Could you check a few things on this model? Use its own coordinates, in mm. A direction names the side the tool comes from. Give positions to 0.01 mm unless a question says otherwise; leave off trailing zeros. Loops run counter-clockwise (first coordinate to the right, second up) from the corner with the lowest first, then second, coordinate; pieces in that order, holes last. Notation, with made-up numbers: M -1,-14.75 L 58,-14.75 A7 ccw 58,-8.75 Z; hole C 81.5,-31.75 d10. An arc over 180 degrees is marked long. Use a Markdown table: item, result. Add a question column.
1) If I drill on line 1 along Z through (x, y) = (1, -6.5); line 2 along Y through (x, z) = (-2.25, -1.5); line 3 along Y through (x, z) = (0.5, -3.5), over which ranges is the centre line in solid material (lowest first)? Write a range as [from, to].
2) Will these pins go through, and if not, where does the flat tip stop? pin 1 Ø3 at (x, y) = (-1.5, 1.5) entering from -Z; pin 2 Ø4 at (y, z) = (3.5, 9) entering from +X; pin 3 Ø4 at (x, z) = (2, -4) entering from -Y; pin 4 Ø2 at (x, y) = (-4.5, 6) entering from -Z.
3) We'd pull the mould along X, two halves only. Please class faces 3 (the conical face through (-3.45, 2.65, 2.83)), 4 (the cylindrical face through (-1.19, 5.37, -0.13)), 5 (the flat face through (-5, 0, -9)): +X half, -X half, draft (parallel to the pull), parting line (faces both ways), or undercut.
4) Which directions (+Z, -Z, +X, -X, +Y, -Y) give clear straight access to the entire face, cutting with the end or side of a thin tool? Please do faces 1 (the cylindrical face through (7.81, 1.73, 11.71)), 2 (the flat face through (1.7, 5.4, 9)).
5) Suppose I cut it at A-A on z = -3.25. List the corners of the cut face in (x, y) for me, and give its area (3 significant figures).
6) Suppose I cut it at B-B on z = 5. List the corners of the cut face in (x, y) for me, and give its area (3 significant figures).
Solid Edge part; units mm, degrees
sketch "Sketch1" plane through (0, 0, 0) normal (0, 0, 1) x (1, 0, 0)
  circle A0 centre (0, 0) radius 5.5
extrude "Ajout_matière_1" add sketch "Sketch1" along normal mid plane 18
sketch "Sketch2" plane through (0, 0, 9) normal (0, 0, 1) x (0, -1, 0)
  circle A0 centre (0, 0) radius 8
extrude "Ajout_matière_3" add sketch "Sketch2" along normal blind 6
sketch "Sketch3" plane through (0, 0, 15) normal (0, 0, 1) x (1, 0, 0)
  circle A0 centre (0, 0) radius 4.2
extrude "Cutout1" cut sketch "Sketch3" against normal up to next and the other way up to next
draft "Dépouille_4" angle 0.7 neutral plane through (0, 0, 15) normal (0, 0, 1) pull direction (0, 0, -1) face at (2.3242, 3.4983, -4.76)
chamfer "Chanfrein_2" distance 0.5 angle 45 1 edges at (0, 8, 15)
properties material "Plastique ABS, haute performance"
Answer block:
| question | item | result |
|---|---|---|
| 1 | line 1 | z = [9, 15] |
| 1 | line 2 | y = [-5.02, -3.78], [3.78, 5.02] |
| 1 | line 3 | y = [-5.48, -4.4], [4.4, 5.48] |
| 2 | pin 1 | passes through |
| 2 | pin 2 | stops at x = 7.86 |
| 2 | pin 3 | stops at y = -5.5 |
| 2 | pin 4 | stops at z = 9 |
| 3 | face 3 | undercut |
| 3 | face 4 | parting line |
| 3 | face 5 | draft |
| 4 | face 1 | +Z, -Z |
| 4 | face 2 | -Z |
| 5 | outline | C 0,0 d11; hole C 0,0 d8.85 |
| 5 | area | 33.6 mm^2 |
| 6 | outline | C 0,0 d11; hole C 0,0 d8.64 |
| 6 | area | 36.3 mm^2 |
